The model under review builds one solid part; all positions refer to its coordinate system, in mm. A direction names the side the tool comes from. Give positions to 0.01 mm unless a question says otherwise; leave off trailing zeros. Loops run counter-clockwise (first coordinate to the right, second up) from the corner with the lowest first, then second, coordinate; pieces in that order, holes last. Notation, with made-up numbers: M 23,16.5 L 71,16.5 A22 ccw 71,40.5 Z; hole C -27.75,44.5 d4. An arc over 180 degrees is marked long. Put each result on its own line as item: value. Start each with the question number.
from build123d import *

# Parameters (mm, degrees)
ESBO_O1_W                = 222
ESBO_O1_H                = 120
RESSALTO_EXTRUS_O1_DEPTH = 6
ESBO_O3_W                = 6
ESBO_O3_H                = 6
CORTE_EXTRUS_O1_DEPTH    = 134.018795664
PADR_O_LINEAR2_COUNT     = 5
PADR_O_LINEAR2_PITCH     = 12


with BuildPart() as part:
    # Esboço1 → Ressalto-extrusão1 (new body)
    with BuildSketch(Plane.XY):
        with Locations((6, -3)):
            Rectangle(ESBO_O1_W, ESBO_O1_H)
    extrude(amount=RESSALTO_EXTRUS_O1_DEPTH)

    # Esboço3 → Corte-extrusão1 (cut, through all)
    with BuildSketch(Plane.XY.offset(6)):
        with Locations((-102, 0)):
            Rectangle(ESBO_O3_W, ESBO_O3_H)
    corte_extrus_o1 = extrude(amount=-CORTE_EXTRUS_O1_DEPTH, mode=Mode.SUBTRACT)

    # Padrão linear2: Corte-extrusão1 ×5
    with Locations(*[(0, i * PADR_O_LINEAR2_PITCH, 0) for i in range(1, PADR_O_LINEAR2_COUNT)]):
        add(corte_extrus_o1, mode=Mode.SUBTRACT)


solid = part.part
(1) Insertion check: pin 1 (1.8 mm diameter, centred on y = 22.5, z = 2.5, fed in from -X). The pin has a flat end and moves straight along its axis. Give the tip position at first contact, or say it passes through.
(2) We need section A-A, the plane y = 48.5. Write out the cut boundary in (x, z), plus the area to 3 significant figures.
(3) For faces 1 (the flat face through (-99, 36, 3)), 2 (the flat face through (4, -2, 0)), list the 3-axis set-ups (+Z, -Z, +X, -X, +Y, -Y) from which the entire face can be reached by the end or side of a thin tool; tool diameter is ignored.
(4) Draft analysis for pull direction Y (two halves, no side actions). For faces 3 (the flat face through (-99, 48, 3)), 4 (the flat face through (-105, 54, 3)), 5 (the flat face through (-99, 0, 3)), 6 (the flat face through (4, 57, 3)), state which applies: +Y half, -Y half, draft (parallel to the pull), parting line (faces both ways), or undercut.
(5) To check wall thickness, follow L1, parallel to X at y = 47, z = 2.9. State the ranges of the line that lie inside material, in increasing order. Write a range as [from, to].
Check sheet entries:
1. pin 1: stops at x = -99
2. outline: M -99,0 L 117,0 L 117,6 L -99,6 Z
2. area: 1,300 mm²
3. face 1: +Z, -Z, -X
3. face 2: -Z, +X, -X, +Y, -Y
4. face 3: undercut
4. face 4: draft
4. face 5: undercut
4. face 6: +Y half
5. L1: x = [-99, 117]
